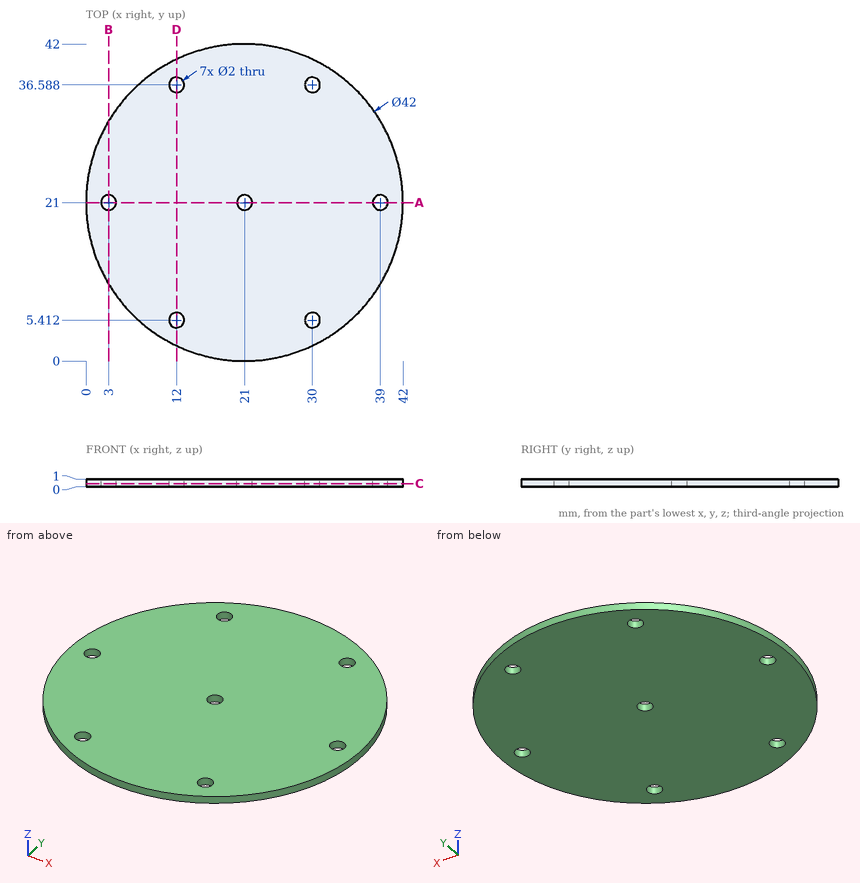
Part print with two shaded views. Sizes in mm from the minimum x, y, z corner. Coordinates: 2 decimals unless noted, no trailing zeros. Write each loop counter-clockwise with the first axis right and the second up, starting at its lowest first coordinate (ties: lowest second). Pieces come first, ordered by that corner, then holes. Notation, with made-up numbers: (61.25, 39) - (91.25, 39) arc R22 cw to (91.25, 64) - close; hole circle Ø10 at (69, -28.75). An arc over 180 degrees is marked (long way). Put each result on its own line as item: value.
1. Band-saw the part on B-B (x = 3). Write the cut outline in (y, z).
Final values:
outline: (10.18, 0) - (20, 0) - (20, 1) - (10.18, 1) - close; (22, 0) - (31.82, 0) - (31.82, 1) - (22, 1) - close
2. Probe line 1 along Y through (x, z) = (12, 0.35) (1 decimal); line 2 along X through (y, z) = (4.5, 0.45) (1 decimal); line 3 along Y through (x, z) = (35, 0.7). List the from-to ranges inside material, lowest first. Write a range as [from, to].
Final values:
line 1: y = [2, 4.4], [6.4, 35.6], [37.6, 40]
line 2: x = [8, 11.6], [12.4, 29.6], [30.4, 34]
line 3: y = [5.35, 36.65]
3. Band-saw the part on D-D (x = 12). Write the cut outline in (y, z).
Final values:
outline: (2.03, 0) - (4.41, 0) - (4.41, 1) - (2.03, 1) - close; (6.41, 0) - (35.59, 0) - (35.59, 1) - (6.41, 1) - close; (37.59, 0) - (39.97, 0) - (39.97, 1) - (37.59, 1) - close
4. Band-saw the part on A-A (y = 21). Write the cut outline in (x, z).
Final values:
outline: (0, 0) - (2, 0) - (2, 1) - (0, 1) - close; (4, 0) - (20, 0) - (20, 1) - (4, 1) - close; (22, 0) - (38, 0) - (38, 1) - (22, 1) - close; (40, 0) - (42, 0) - (42, 1) - (40, 1) - close
5. Band-saw the part on C-C (z = 0.4). Write the cut outline in (x, y).
Final values:
outline: circle Ø42 at (21, 21); hole circle Ø2 at (3, 21); hole circle Ø2 at (12, 5.41); hole circle Ø2 at (12, 36.59); hole circle Ø2 at (21, 21); hole circle Ø2 at (30, 5.41); hole circle Ø2 at (30, 36.59); hole circle Ø2 at (39, 21)
